```python
from build123d import *

# Parameters (mm, degrees)
SKETCH_1_W          = 53
SKETCH_1_H          = 38
SKETCH_1_W_2        = 45
SKETCH_1_H_2        = 30
EXTRUDE_1_DEPTH     = 6
SKETCH_2_R          = 1.5
CUT_EXTRUDE_1_DEPTH = 59
SKETCH_4_W          = 53
SKETCH_4_H          = 2
EXTRUDE_1_2_DEPTH   = 6
SKETCH_5_R          = 1.5
CUT_EXTRUDE_3_DEPTH = 59
SKETCH_11_W         = 53
SKETCH_11_H         = 4
CUT_EXTRUDE_5_DEPTH = 10
SKETCH_12_W         = 53
SKETCH_12_H         = 30
CUT_EXTRUDE_6_DEPTH = 10
SKETCH_13_R         = 1.25
CUT_EXTRUDE_7_DEPTH = 10
SKETCH_14_W         = 10
SKETCH_14_H         = 6
CUT_EXTRUDE_8_DEPTH = 10


with BuildPart() as part:
    # 草图1 → Extrude 1 (new body)
    with BuildSketch(Plane.XY):
        Rectangle(SKETCH_1_W, SKETCH_1_H)
        Rectangle(SKETCH_1_W_2, SKETCH_1_H_2, mode=Mode.SUBTRACT)
    extrude(amount=EXTRUDE_1_DEPTH)

    # 草图2 → 切除-拉伸1 (cut)
    with BuildSketch(Plane.ZY.offset(26.5)):
        with Locations((3.5, 9)):
            Circle(SKETCH_2_R)
        with Locations((3.5, -9)):
            Circle(SKETCH_2_R)
    extrude(amount=-CUT_EXTRUDE_1_DEPTH, mode=Mode.SUBTRACT)

    # 草图4 → Extrude 1 2 (add)
    with BuildSketch(Plane(origin=(0, 0, 0), x_dir=(-1, 0, 0), z_dir=(0, 0, -1))):
        with Locations((0, -20)):
            Rectangle(SKETCH_4_W, SKETCH_4_H)
    extrude(amount=-EXTRUDE_1_2_DEPTH)

    # 草图5 → 切除-拉伸3 (cut)
    with BuildSketch(Plane(origin=(0, 0, 0), x_dir=(-1, 0, 0), z_dir=(0, 0, -1))):
        with Locations((12, -18)):
            Circle(SKETCH_5_R)
        with Locations((-12, -18)):
            Circle(SKETCH_5_R)
    extrude(amount=-CUT_EXTRUDE_3_DEPTH, mode=Mode.SUBTRACT)

    # 草图11 → 切除-拉伸5 (cut)
    with BuildSketch(Plane.XY.offset(6)):
        with Locations((0, 17)):
            Rectangle(SKETCH_11_W, SKETCH_11_H)
    extrude(amount=-CUT_EXTRUDE_5_DEPTH, mode=Mode.SUBTRACT)

    # 草图12 → 切除-拉伸6 (cut)
    with BuildSketch(Plane.XY.offset(6)):
        Rectangle(SKETCH_12_W, SKETCH_12_H)
    extrude(amount=-CUT_EXTRUDE_6_DEPTH, mode=Mode.SUBTRACT)

    # 草图13 → 切除-拉伸7 (cut)
    with BuildSketch(Plane.XZ.offset(21)):
        with Locations(Location((8, 3, 0), (0, 0, 270))):
            Circle(SKETCH_13_R)
        with Locations(Location((-8, 3, 0), (0, 0, 270))):
            Circle(SKETCH_13_R)
    extrude(amount=-CUT_EXTRUDE_7_DEPTH, mode=Mode.SUBTRACT)

    # 草图14 → 切除-拉伸8 (cut)
    with BuildSketch(Plane(origin=(0, 0, 0), x_dir=(-1, 0, 0), z_dir=(0, 0, -1))):
        with Locations((21.5, -18)):
            Rectangle(SKETCH_14_W, SKETCH_14_H)
        with Locations((-21.5, -18)):
            Rectangle(SKETCH_14_W, SKETCH_14_H)
    extrude(amount=-CUT_EXTRUDE_8_DEPTH, mode=Mode.SUBTRACT)


solid = part.part
```
For this review, take the finished solid that the model builds, in its own axes (mm). Give positions to 0.01 mm unless a question says otherwise; leave off trailing zeros. Write each loop counter-clockwise with the first axis right and the second up, starting at its lowest first coordinate (ties: lowest second). Pieces come first, ordered by that corner, then holes. Notation, with made-up numbers: M 39,41 L 74,41 A25 ccw 74,58 Z; hole C 17.25,32 d11. An arc over 180 degrees is marked long. Answer as CSV lines item,"result".
1. Wall thickness on line 1 (X direction, y = -20.35, z = 3.1); line 2 (X direction, y = -20.5, z = 2.2); line 3 (X direction, y = -17, z = 3): over which ranges is each line inside the solid? List them lowest first.
Findings:
line 1,"x = -16.5 to -9.25, -6.75 to 6.75, 9.25 to 16.5"
line 2,"x = -16.5 to -8.96, -7.04 to 7.04, 8.96 to 16.5"
line 3,"x = -16.5 to -13.12, -10.88 to -9.25, -6.75 to 6.75, 9.25 to 10.88, 13.12 to 16.5"
2. Consider section D-D, the plane x = 12. Write out the cut boundary in (y, z), then the cut area to 3 significant figures.
Findings:
outline,"M -21,0 L -19.5,0 L -19.5,6 L -21,6 Z; M -16.5,0 L -15,0 L -15,6 L -16.5,6 Z"
area,"18.0 mm2"
3. Draft analysis for pull direction Z (two halves, no side actions). For faces 1 (the flat face through (0, -21, 3)), 2 (the flat face through (0, -18, 6)), 3 (the cylindrical face through (7.521, -18.042, 1.845)), state which applies: +Z half, -Z half, draft (parallel to the pull), parting line (faces both ways), or undercut.
Findings:
face 1,"draft"
face 2,"+Z half"
face 3,"undercut"
4. Consider section A-A, the plane x = -8. Write out the cut boundary in (y, z).
Findings:
outline,"M -21,0 L -15,0 L -15,1.75 L -21,1.75 Z; M -21,4.25 L -15,4.25 L -15,6 L -21,6 Z"
5. Consider section C-C, the plane z = 3.9. Write out the cut boundary in (x, y), then the cut area to 3 significant figures.
Findings:
outline,"M -16.5,-21 L -8.87,-21 L -8.87,-15 L -16.5,-15 Z; M -7.13,-21 L 7.13,-21 L 7.13,-15 L -7.13,-15 Z; M 8.87,-21 L 16.5,-21 L 16.5,-15 L 8.87,-15 Z; hole C -12,-18 d3; hole C 12,-18 d3"
area,"163 mm2"
6. Consider section B-B, the plane y = -18. Write out the cut boundary in (x, z).
Findings:
outline,"M -16.5,0 L -13.5,0 L -13.5,6 L -16.5,6 Z; M -10.5,0 L 10.5,0 L 10.5,6 L -10.5,6 Z; M 13.5,0 L 16.5,0 L 16.5,6 L 13.5,6 Z; hole C -8,3 d2.5; hole C 8,3 d2.5"
7. For pin 1 (1.8 mm diameter, centred on x = 12, y = -18, fed in from +Z), flat-tipped, find the tip position at first contact; note if it passes through.
Findings:
pin 1,"passes through"
